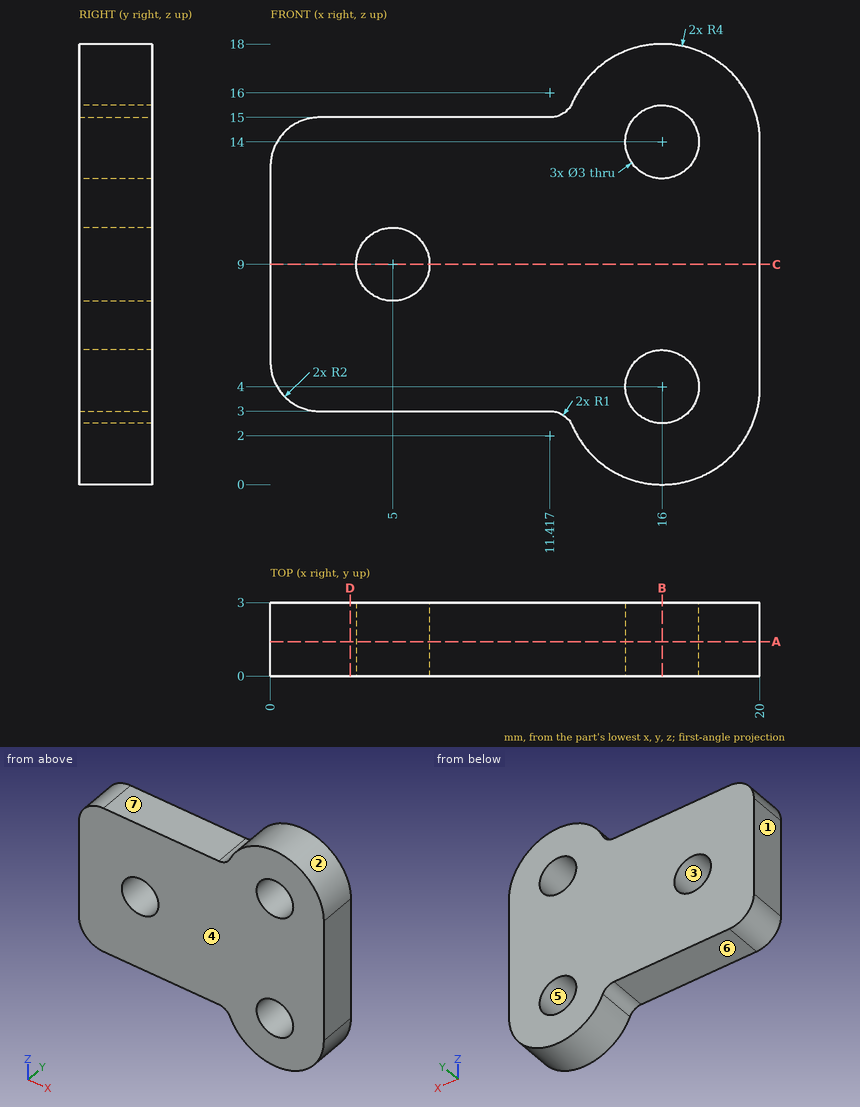
Geometry: see drawing. Coordinates: mm, zero at the bounding-box minimum. A direction names the side the tool comes from. Give positions to 0.01 mm unless a question says otherwise; leave off trailing zeros. Order: outer loops, then holes, each group sorted by start corner. A loop starts at its lowest first (then second) coordinate and runs counter-clockwise, first axis right, second up. Notation, with made-up numbers: (50.5, 73) -> (100.5, 73) arc R27 ccw to (100.5, 93) -> close; hole circle Ø9 at (15, -0.5). An arc over 180 degrees is marked (long way). Write each question's results on one line, items separated by ' | '. Start each with the question number.
1) Set-up query: the marked faces 5, 6 and 7. Return all of +Z, -Z, +X, -X, +Y, -Y with unobstructed straight access to the full face (end or side cutting, diameter ignored); none if empty.
2) Section D-D (x = 3.25). Return loops of the section in (y, z), then the cut area to 3 significant figures.
3) Draft query along X for the marked faces 1, 2, 3 and 4. Return one class per face: pulls with the +X half, pulls with the -X half, needs draft (parallel to the pull), parting line crosses it, or undercut.
4) Section A-A (y = 1.4). Return loops of the section in (x, z), then the cut area to 3 significant figures.
5) Line query: line 1 (Z direction, x = 16, y = 1.15); line 2 (Z direction, x = 5, y = 1.75); line 3 (Z direction, x = 7.5, y = 1.2). Output: solid intervals per line, ascending. Write a range as from..to.
6) First-contact query: pin 1 (2.5 mm diameter, centred on x = 16, z = 14, fed in from -Y); pin 2 (1.5 mm diameter, centred on y = 1, z = 2.5, fed in from +X); pin 3 (1 mm diameter, centred on x = 8, z = 11.5, fed in from -Y); pin 4 (1.5 mm diameter, centred on x = 6, y = 1, fed in from +Z). Flat tips, straight axial feed; report the tip coordinate or a pass-through.
7) Section C-C (z = 9). Return loops of the section in (x, y).
8) Section B-B (x = 16). Return loops of the section in (y, z), then the cut area to 3 significant figures.
Calculated:
1) face 5: +Y, -Y | face 6: -Z, -X, +Y, -Y | face 7: +Z, -X, +Y, -Y
2) outline: (0, 3) -> (3, 3) -> (3, 15) -> (0, 15) -> close | area: 36.0 mm2
3) face 1: pulls with the -X half | face 2: parting line crosses it | face 3: undercut | face 4: needs draft
4) outline: (0, 5) arc R2 ccw to (2, 3) -> (11.42, 3) arc R1 cw to (12.33, 2.4) arc R4 ccw to (20, 4) -> (20, 14) arc R4 ccw to (12.33, 15.6) arc R1 cw to (11.42, 15) -> (2, 15) arc R2 ccw to (0, 13) -> close; hole circle Ø3 at (5, 9); hole circle Ø3 at (16, 4); hole circle Ø3 at (16, 14) | area: 252 mm2
5) line 1: 0..2.5, 5.5..12.5, 15.5..18 | line 2: 3..7.5, 10.5..15 | line 3: 3..15
6) pin 1: through | pin 2: x = 19.93 | pin 3: y = 0 | pin 4: z = 15
7) outline: (0, 0) -> (3.5, 0) -> (3.5, 3) -> (0, 3) -> close; (6.5, 0) -> (20, 0) -> (20, 3) -> (6.5, 3) -> close
8) outline: (0, 0) -> (3, 0) -> (3, 2.5) -> (0, 2.5) -> close; (0, 5.5) -> (3, 5.5) -> (3, 12.5) -> (0, 12.5) -> close; (0, 15.5) -> (3, 15.5) -> (3, 18) -> (0, 18) -> close | area: 36.0 mm2
